Could you check a few things on this drawing? It's one solid part, dimensions in mm from its lowest x, y, z. Give positions to 0.01 mm unless a question says otherwise; leave off trailing zeros. Loops run counter-clockwise (first coordinate to the right, second up) from the corner with the lowest first, then second, coordinate; pieces in that order, holes last. Notation, with made-up numbers: M -29.75,12.25 L 10.25,12.25 A6 ccw 10.25,19.25 Z; hole C 31,38.5 d1. An arc over 180 degrees is marked long. Answer in a Markdown table with one row per item. Add a question column.
1. I need wall thicknesses on line 1 along Z through (x, y) = (96, 52); line 2 along Y through (x, z) = (216, 54); line 3 along X through (y, z) = (146, 52). Which ranges of each line are inside material? Lowest first, please. Write a range as from..to.
2. If we section it at D-D on z = 79.5: List the corners of the cut face in (x, y) for me.
3. Thinking about a two-plate mould opening in Z: for the marked faces 1 and 2, which applies, released by +Z, released by -Z, zero draft, split by the parting line, or undercut?
4. If we section it at B-B on x = 113.5: List the corners of the cut face in (y, z) for me, then the cut area to 3 significant figures.
5. If we section it at C-C on y = 35.5: List the corners of the cut face in (x, z) for me, then the cut area to 3 significant figures.
6. I'm going to push flat-ended pins straight in: pin 1 Ø1.5 at (y, z) = (144, 93) entering from +X; pin 2 Ø4 at (x, z) = (158.5, 48.5) entering from -Y; pin 3 Ø6 at (x, z) = (143.5, 42) entering from -Y. Where does each tip first touch, or does it pass through?
7. If we section it at A-A on z = 52.45: List the corners of the cut face in (x, y) for me.
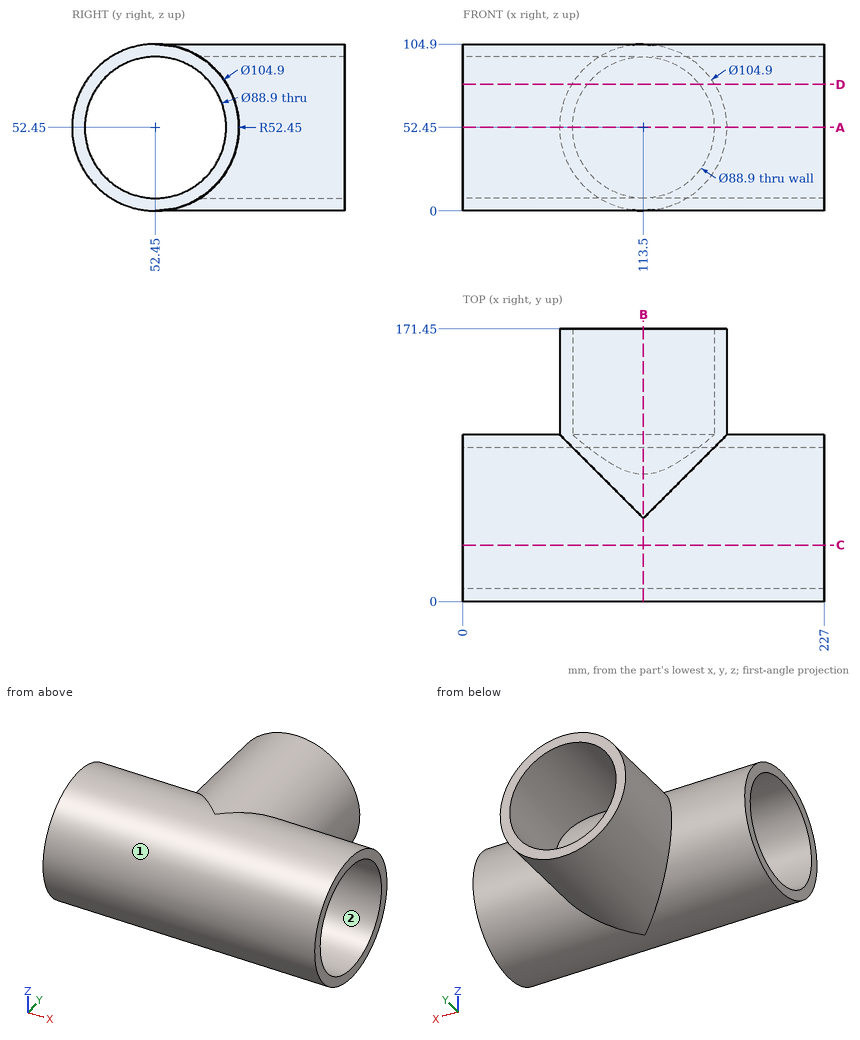
Results:
| question | item | result |
|---|---|---|
| 1 | line 1 | 0..8, 96.9..104.9 |
| 1 | line 2 | 0.02..8.03, 96.87..104.88 |
| 1 | line 3 | 61.05..69.05, 157.95..165.95 |
| 2 | outline | M 0,7.51 L 227,7.51 L 227,17.18 L 0,17.18 Z; M 0,87.72 L 227,87.72 L 227,97.39 L 158.44,97.39 L 158.44,171.45 L 148.77,171.45 L 148.77,97.39 L 78.23,97.39 L 78.23,171.45 L 68.56,171.45 L 68.56,97.39 L 0,97.39 Z |
| 3 | face 1 | split by the parting line |
| 3 | face 2 | undercut |
| 4 | outline | M 52.45,0 L 171.45,0 L 171.45,8 L 80.29,8 A52.45 ccw 80.29,96.9 L 171.45,96.9 L 171.45,104.9 L 52.45,104.9 A52.45 ccw Z; hole C 52.45,52.45 d88.9 |
| 4 | area | 4,040 mm2 |
| 5 | outline | M 0,2.81 L 227,2.81 L 227,11.36 L 0,11.36 Z; M 0,93.54 L 227,93.54 L 227,102.09 L 0,102.09 Z |
| 5 | area | 3,880 mm2 |
| 6 | pin 1 | x = 147.66 |
| 6 | pin 2 | y = 0.04 |
| 6 | pin 3 | y = 0.53 |
| 7 | outline | M 0,0 L 227,0 L 227,8 L 0,8 Z; M 0,96.9 L 227,96.9 L 227,104.9 L 165.95,104.9 L 165.95,171.45 L 157.95,171.45 L 157.95,104.9 L 69.05,104.9 L 69.05,171.45 L 61.05,171.45 L 61.05,104.9 L 0,104.9 Z |
